Print and shaded views of the part. All mm, measured from the part's lowest x, y and z. A direction names the side the tool comes from. Round coordinates to 2 decimals unless told otherwise and drop trailing zeros. Write each loop counter-clockwise with the first axis right and the second up, starting at its lowest first coordinate (ties: lowest second). Pieces come first, ordered by that corner, then holes. Notation, with made-up numbers: (65.25, -13) - (91.25, -13) arc R30 ccw to (91.25, 24) - close; hole circle Ø6 at (75, 72). An arc over 180 degrees is marked (long way). Put each result on its own line as item: value. Start each with the question number.
Item 1: Cut at D-D (z = 3.5). Give the cut face in (x, y).
Item 2: Drill centre lines: line 1 (Y direction, x = 29.2, z = 15); line 2 (Z direction, x = 2.25, y = 101). Where is each one in solid material? Low to high. Write a range as from..to.
Item 3: Pin check, flat tips, straight feed: pin 1 Ø1.5 at (x, z) = (11, 26.5) entering from +Y; pin 2 Ø2 at (x, y) = (23.5, 112) entering from -Z. Stop position of each tip, or through.
Item 4: Cut at A-A (z = 15). Give the cut face in (x, y).
Item 5: Mould opens along Z. For the marked faces 1, 2 and 3 say: released by +Z, released by -Z, zero draft, split by the parting line, or undercut.
Item 6: 3-axis set-ups, long thin cutter, end or side, ignore diameter. For the marked faces 4 and 5: which of +Z, -Z, +X, -X, +Y, -Y reach the whole face in a straight line?
Item 7: Cut at B-B (y = 15). Give the cut face in (x, z).
Item 8: Cut at C-C (x = 6). Give the cut face in (y, z), and give its area (3 significant figures).
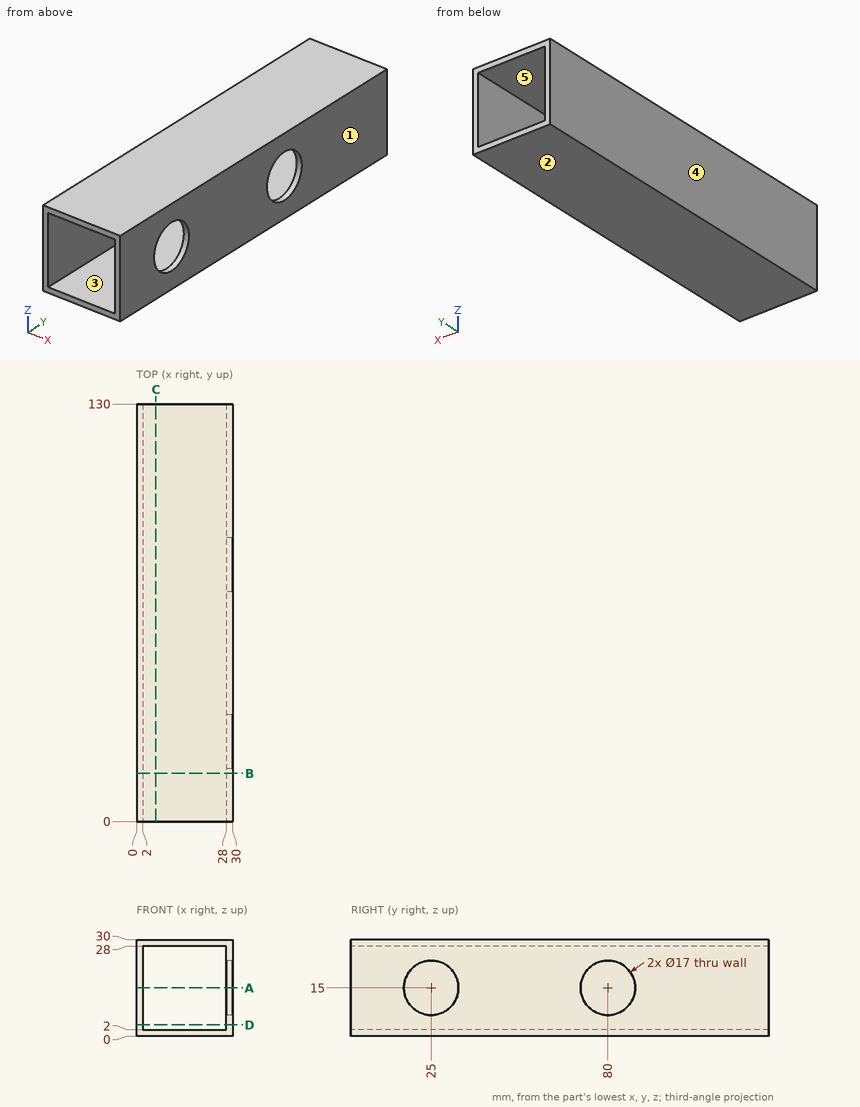
Output values:
1. outline: (0, 0) - (2, 0) - (2, 130) - (0, 130) - close; (28, 0) - (30, 0) - (30, 130) - (28, 130) - close
2. line 1: 0..16.5, 33.5..71.5, 88.5..130
2. line 2: 0..2, 28..30
3. pin 1: through
3. pin 2: z = 0
4. outline: (0, 0) - (2, 0) - (2, 130) - (0, 130) - close; (28, 0) - (30, 0) - (30, 16.5) - (28, 16.5) - close; (28, 33.5) - (30, 33.5) - (30, 71.5) - (28, 71.5) - close; (28, 88.5) - (30, 88.5) - (30, 130) - (28, 130) - close
5. face 1: zero draft
5. face 2: released by -Z
5. face 3: undercut
6. face 4: +Z, -Z, -X, +Y, -Y
6. face 5: +Y, -Y
7. outline: (0, 0) - (30, 0) - (30, 30) - (0, 30) - close; hole (2, 2) - (28, 2) - (28, 28) - (2, 28) - close
8. outline: (0, 0) - (130, 0) - (130, 2) - (0, 2) - close; (0, 28) - (130, 28) - (130, 30) - (0, 30) - close
8. area: 520 mm2
